Autodesk Inventor part; units mm, degrees
ref_plane "YZ Plane" through (0, 0, 0) normal (1, 0, 0) x (0, 1, 0)
ref_plane "XZ Plane" through (0, 0, 0) normal (0, 1, 0) x (-1, 0, 0)
ref_plane "XY Plane" through (0, 0, 0) normal (0, 0, 1) x (1, 0, 0)
sketch "Sketch1" plane through (0, 0, 0) normal (0, 1, 0) x (-1, 0, 0)
  line L0 (19.558, 10.033) -> (-19.558, 10.033)
  line L1 (-19.558, 10.033) -> (-19.558, -10.033)
  line L2 (-19.558, -10.033) -> (19.558, -10.033)
  line L3 (19.558, -10.033) -> (19.558, 10.033)
  line L4 (19.558, 10.033) -> (-19.558, -10.033) construction
  line L5 (-19.558, 10.033) -> (19.558, -10.033) construction
  line L6 (25.908, 16.383) -> (-25.908, 16.383)
  line L7 (-25.908, 16.383) -> (-25.908, -16.383)
  line L8 (-25.908, -16.383) -> (25.908, -16.383)
  line L9 (25.908, -16.383) -> (25.908, 16.383)
  line L10 (25.908, 16.383) -> (-25.908, -16.383) construction
  line L11 (-25.908, 16.383) -> (25.908, -16.383) construction
  point P0 (0, 0)
  dimension "d0" = 20.066
  dimension "d1" = 39.116
  dimension "d2" = 6.35
  dimension "d3" = 6.35
extrude "Extrusion1" add sketch "Sketch1" against normal blind 12.7
sketch "Sketch2" plane through (0, 0, 0) normal (0, 1, 0) x (1, 0, 0)
  line L0 (25.908, -16.383) -> (-25.908, -16.383)
  line L1 (-25.908, 16.383) -> (25.908, 16.383)
  line L2 (-25.908, -16.383) -> (25.908, -16.383)
  line L3 (25.908, -16.383) -> (25.908, 16.383)
  line L4 (25.908, 16.383) -> (-25.908, 16.383)
  line L5 (-25.908, 16.383) -> (-25.908, -16.383)
  point P0 (0, 0)
extrude "Extrusion2" add sketch "Sketch2" along normal blind 6.35
fillet "Fillet1" radius 6.35 4 edges at (0, 6.35, 16.383) (25.908, 6.35, 0) (0, 6.35, -16.383) (-25.908, 6.35, 0)
fillet "Fillet2" radius 6.35 8 edges at (24.0481, 4.4901, 14.5231) (25.908, -6.35, 16.383) (24.0481, 4.4901, -14.5231) (25.908, -6.35, -16.383) (-24.0481, 4.4901, 14.5231) (-25.908, -6.35, 16.383) (-24.0481, 4.4901, -14.5231) (-25.908, -6.35, -16.383)
sketch "Sketch3" plane through (-19.558, -12.7, 16.383) normal (0, 0, 1) x (1, 0, 0)
  line L0 (0, 0) -> (-6.35, 0) construction
  line L1 (45.466, 12.7) -> (39.116, 12.7) construction
  line L2 (0, 0) -> (39.116, 12.7) construction
  line L3 (39.116, 12.7) -> (39.116, 0) construction
  line L4 (0, 19.05) -> (0, 12.7) construction
  line L5 (39.116, 0) -> (0, 12.7) construction
  point P0 (19.558, 12.7)
  point P1 (19.558, 6.35)
hole "Hole1" at (0, -6.35, 16.383) direction (0, 0, -1) diameter 5.1054 end through all
equation "\"d0\" = width + 2 * printerError"
equation "\"d1\" = length + 2 * printerError"
equation "\"d2\" = wallThickness"
equation "\"d3\" = wallThickness"
equation "\"d4\" = heightFromTop"
equation "\"d6\" = thicknessAboveTopOfPost"
equation "\"width\" = 19.05"
equation "\"length\" = 38.1"
equation "\"heightFromTop\" = 12.7"
equation "\"thicknessAboveTopOfPost\" = 6.35"
equation "\"printerError\" = 0.508"
equation "\"wallThickness\" = 6.35"
properties part number "PostCap"
Model file for the job. Use its own axes, mm. A direction names the side the tool comes from. Give positions to 0.01 mm unless a question says otherwise; leave off trailing zeros. Write each loop counter-clockwise with the first axis right and the second up, starting at its lowest first coordinate (ties: lowest second). Pieces come first, ordered by that corner, then holes. Notation, with made-up numbers: (78, -8) - (116, -8) arc R21 ccw to (116, 19) - close; hole circle Ø2 at (19, 75.5). An arc over 180 degrees is marked (long way). Answer as CSV lines item,"result".
1. Two-plate mould, pull along Z, no slides. Class faces 3 (the face through (-0.27, 4.44, 14.57)), 4 (the face through (-0.767, -8.785, -13.252)), 5 (the face through (-19.558, -6, 0)): +Z half, -Z half, draft (parallel to the pull), parting line (faces both ways), or undercut.
Responses:
face 3,"+Z half"
face 4,"draft"
face 5,"undercut"
2. 3-axis set-ups, long thin cutter, end or side, ignore diameter. For faces 1 (the face through (24, 4.54, -0.14)), 2 (the face through (19.558, -6, 0)): which of +Z, -Z, +X, -X, +Y, -Y reach the whole face in a straight line?
Responses:
face 1,"+Z, -Z, +X, +Y"
face 2,"-Y"
3. Band-saw the part on A-A (y = -6.35). Write the cut outline in (x, z), and give its area (3 significant figures).
Responses:
outline,"(-25.91, -10.03) arc R6.35 ccw to (-19.56, -16.38) - (-2.55, -16.38) - (-2.55, -10.03) - (-19.56, -10.03) - (-19.56, 10.03) - (-2.55, 10.03) - (-2.55, 16.38) - (-19.56, 16.38) arc R6.35 ccw to (-25.91, 10.03) - close; (2.55, -16.38) - (19.56, -16.38) arc R6.35 ccw to (25.91, -10.03) - (25.91, 10.03) arc R6.35 ccw to (19.56, 16.38) - (2.55, 16.38) - (2.55, 10.03) - (19.56, 10.03) - (19.56, -10.03) - (2.55, -10.03) - close"
area,"813 mm2"
4. Band-saw the part on D-D (x = -15.5). Write the cut outline in (y, z), and give its area (3 significant figures).
Responses:
outline,"(-12.7, -16.38) - (0, -16.38) arc R6.35 ccw to (6.35, -10.03) - (6.35, 10.03) arc R6.35 ccw to (0, 16.38) - (-12.7, 16.38) - (-12.7, 10.03) - (0, 10.03) - (0, -10.03) - (-12.7, -10.03) - close"
area,"352 mm2"
5. Drill centre lines: L1, parallel to Z at x = 6, y = -8.5; L2, parallel to X at y = -1, z = -8.5; L3, parallel to X at y = -6.35, z = -13.5. Where is each one in solid material? Low to high. Write a range as [from, to].
Responses:
L1,"z = [-16.38, -10.03], [10.03, 16.38]"
L2,"x = [-25.91, -19.56], [19.56, 25.91]"
L3,"x = [-24.88, -2.55], [2.55, 24.88]"
6. Band-saw the part on B-B (x = 0). Write the cut outline in (y, z).
Responses:
outline,"(-12.7, -16.38) - (-8.9, -16.38) - (-8.9, -10.03) - (-12.7, -10.03) - close; (-12.7, 10.03) - (-8.9, 10.03) - (-8.9, 16.38) - (-12.7, 16.38) - close; (-3.8, -16.38) - (0, -16.38) arc R6.35 ccw to (6.35, -10.03) - (6.35, 10.03) arc R6.35 ccw to (0, 16.38) - (-3.8, 16.38) - (-3.8, 10.03) - (0, 10.03) - (0, -10.03) - (-3.8, -10.03) - close"
7. Band-saw the part on C-C (z = -2). Write the cut outline in (x, y).
Responses:
outline,"(-25.91, -12.7) - (-19.56, -12.7) - (-19.56, 0) - (19.56, 0) - (19.56, -12.7) - (25.91, -12.7) - (25.91, 0) arc R6.35 ccw to (19.56, 6.35) - (-19.56, 6.35) arc R6.35 ccw to (-25.91, 0) - close"
